from build123d import *

# Parameters (mm, degrees)
F1_DEPTH = 25.4
F3_R     = 8.4043984654
F4_DEPTH = 50.8


with BuildPart() as f1:
    # F0 (on Front) → F1 (new body)
    with BuildSketch(Plane.XZ):
        Polygon((20.0516469777, 0), (0, 0), (26.3161629428, 43.4522676965), (39.4742444142, 65.1784015448), (37.6082088482, 66.6415809447), (-2.7521864977, 0), (-11.9916703552, 0), (-11.9916703552, -24.3765115738), (20.0516469777, -24.3765115738), align=None)
    extrude(amount=F1_DEPTH)

    # F1_face (on face) → F2 (revolve)
    with BuildSketch(Plane(origin=(6.7718176649, -25.4, -3.6801313591), x_dir=(1, 0, 0), z_dir=(0, -1, 0))):
        Polygon((13.2798293128, 3.6801313591), (-6.7718176649, 3.6801313591), (32.7024267493, 68.8585329039), (30.8363911833, 70.3217123039), (-9.5240041626, 3.6801313591), (-18.7634880201, 3.6801313591), (-18.7634880201, -20.6963802146), (13.2798293128, -20.6963802146), align=None)
    revolve(axis=Axis((-11.9916703552, -25.4, -12.1882557869), (0, 0, 1)))

    # F3 (on face) → F4 (cut)
    with BuildSketch(Plane(origin=(0, 0, -24.3765115738), x_dir=(1, 0, 0), z_dir=(0, 0, -1))):
        with Locations((-8.7055349723, 25.3879558295)):
            Circle(F3_R)
    extrude(amount=-F4_DEPTH, mode=Mode.SUBTRACT)


solid = f1.part
Verification items for the finished model (mm, model axes). A direction names the side the tool comes from. Coordinates: 2 decimals unless noted, no trailing zeros. Order: outer loops, then holes, each group sorted by start corner. A loop starts at its lowest first (then second) coordinate and runs counter-clockwise, first axis right, second up. Notation, with made-up numbers: M 85.5,43 L 105.5,43 A27 cw 105.5,79 Z; hole C 15.25,19.25 d7. An arc over 180 degrees is marked long. One line per item, written item: value. Start each with the question number.
Item 1: Gauge pin test, flat ends, axial feed: pin 1 (4 mm diameter, centred on x = 11, z = -11, fed in from +Y); pin 2 (6 mm diameter, centred on x = -44.5, z = 39, fed in from +Y); pin 3 (15 mm diameter, centred on x = -8.71, y = -25.39, fed in from -Z); pin 4 (6 mm diameter, centred on x = -37, z = 33, fed in from +Y). Record the tip position at first contact, or that the pin passes through.
Item 2: Sectioned sample at C-C (z = -12). Enter the section's corners in (x, y).
Item 3: Scan lines: probe 1 along Z at (x, y) = (3, -3.5); probe 2 along Z at (x, y) = (-16, -18); probe 3 along Z at (x, y) = (6.5, -40). Record each from-to range of solid material in increasing order.
Item 4: Mould release check, pull along Z, two halves, no side actions. Record for faces 1 (the flat face through (-20, -25, -24.377)), 2 (the conical face through (-32.14, -24.513, 18.045)), 3 (the flat face through (-12, -39, 0)), 4 (the cylindrical face through (-0.69, -27.91, -10.36)): released by +Z, released by -Z, zero draft, split by the parting line, or undercut.
Item 5: Sectioned sample at B-B (z = 61). Enter the section's corners in (x, y), then the cut area to 3 significant figures.
Item 6: Access from +Z, -Z, +X, -X, +Y, -Y to the whole of each face (thin tool, end or side, straight path). Record for faces 5 (the flat face through (20.052, -13, -12)), 6 (the conical face through (-35.05, -28.24, 18.56)), 7 (the flat face through (14, 0, -12)), 8 (the flat face through (-18, -27, 0)).
Item 7: Sectioned sample at A-A (z = 30). Enter the section's corners in (x, y), then the cut area to 3 significant figures.
Conclusion:
1. pin 1: stops at y = 0
1. pin 2: stops at y = -4.41
1. pin 3: passes through
1. pin 4: stops at y = -1.26
2. outline: M 7.54,0 A32.04 ccw long 20.05,-25.4 L 20.05,0 Z; hole C -8.71,-25.39 d16.81
3. probe 1: z = -24.38 to 0, 4.95 to 9.5, 24.02 to 28.57
3. probe 2: z = -24.38 to 0
3. probe 3: z = -24.38 to 0, 19.1 to 23.65
4. face 1: released by -Z
4. face 2: released by +Z
4. face 3: undercut
4. face 4: zero draft
5. outline: M 34.19,-9.22 A48.94 ccw long 36.94,-25.4 L 36.94,0 L 34.19,0 Z; hole C -11.99,-25.4 d92.37
5. area: 862 mm^2
6. face 5: -Z, +X, +Y, -Y
6. face 6: none
6. face 7: -Z, +X, +Y
6. face 8: +Z
7. outline: M 15.42,-12.81 A30.16 ccw long 18.17,-25.4 L 18.17,0 L 15.42,0 Z; hole C -11.99,-25.4 d54.82
7. area: 544 mm^2
